Autodesk Inventor part; units mm, degrees
ref_plane "YZ Plane" through (0, 0, 0) normal (1, 0, 0) x (0, 1, 0)
ref_plane "XZ Plane" through (0, 0, 0) normal (0, 1, 0) x (-1, 0, 0)
ref_plane "XY Plane" through (0, 0, 0) normal (0, 0, 1) x (1, 0, 0)
sketch "Sketch1" plane through (0, 0, 0) normal (0, 0, 1) x (1, 0, 0)
  line L0 (-33.5517, 0) -> (33.5517, 0)
  line L1 (0, 0) -> (0, 2.95)
  line L2 (0, 2.95) -> (1, 2.95)
  line L3 (1, 2.95) -> (1, 2.5)
  line L4 (1, 2.5) -> (6.1, 2.5)
  arc A0 (8.6, 0) -> (6.1, 2.5) centre (6.1, 0) ccw
  line L5 (8.6, 0) -> (0, 0)
  dimension "d1" = 2.95
  dimension "d2" = 1
  dimension "d3" = 5
  dimension "d4" = 8.6
  dimension "d5" = 2.5
revolve "Revolution1" add sketch "Sketch1" angle 360 about axis through (-33.5517, 0, 0) along (1, 0, 0)
sketch "Sketch2" plane through (0, 0, 0) normal (-1, 0, 0) x (0, 0, 1)
  circle A0 centre (0, 0) radius 2.95
  line L0 (-0.25, 1.52) -> (0.25, 1.52)
  line L1 (0.25, 1.52) -> (0.25, 1.02)
  line L2 (0.25, 1.02) -> (-0.25, 1.02)
  line L3 (-0.25, 1.02) -> (-0.25, 1.52)
  line L4 (-0.25, -1.02) -> (0.25, -1.02)
  line L5 (0.25, -1.02) -> (0.25, -1.52)
  line L6 (0.25, -1.52) -> (-0.25, -1.52)
  line L7 (-0.25, -1.52) -> (-0.25, -1.02)
  line L8 (-0.25, 1.27) -> (0.25, 1.27) construction
  line L9 (-0.25, -1.27) -> (0.25, -1.27) construction
  point P0 (0, 1.52)
  point P1 (0, -1.02)
  dimension "d7" = 0.5
  dimension "d8" = 0.5
  dimension "d9" = 1.27
  dimension "d10" = 1.27
extrude "Extrusion1" add sketch "Sketch2" along normal blind 22.6 contours L0 L1 L2 L3 | L4 L5 L6 L7
sketch "Sketch4" plane through (0, 0, 0) normal (-1, 0, 0) x (0, 0, 1)
  line L0 (-0.25, 1.52) -> (0.25, 1.52)
  circle A0 centre (0, 0) radius 2.95
  circle A1 centre (0, 0) radius 2.5
  line L1 (-1.566, 2.5) -> (1.566, 2.5)
  point P0 (0, 2.5)
extrude "Extrusion2" cut sketch "Sketch4" against normal through all contours L1 A0 picked at (-0.846, 2.5951)
sketch "Sketch3" plane through (-22.6, 0, 0) normal (-1, 0, 0) x (0, 0, 1)
  line L0 (0.25, 1.52) -> (0.25, 1.02)
  line L1 (-0.25, 1.52) -> (0.25, 1.52)
  line L2 (-0.25, 1.02) -> (-0.25, 1.52)
  line L3 (0.25, 1.02) -> (-0.25, 1.02)
  line L4 (0.25, -1.02) -> (0.25, -1.52)
  line L5 (-0.25, -1.02) -> (0.25, -1.02)
  line L6 (-0.25, -1.52) -> (-0.25, -1.02)
  line L7 (0.25, -1.52) -> (-0.25, -1.52)
  point P0 (0, 0)
  point P1 (0, 1.27)
  point P2 (0, -1.27)
  point P3 (-0.25, 1.27)
  point P4 (-0.25, -1.27)
equation "\"d10\" = d9"
equation "\"Lead_solder\" = 1"
properties part number "LED 5mm Red height 1-20mm"
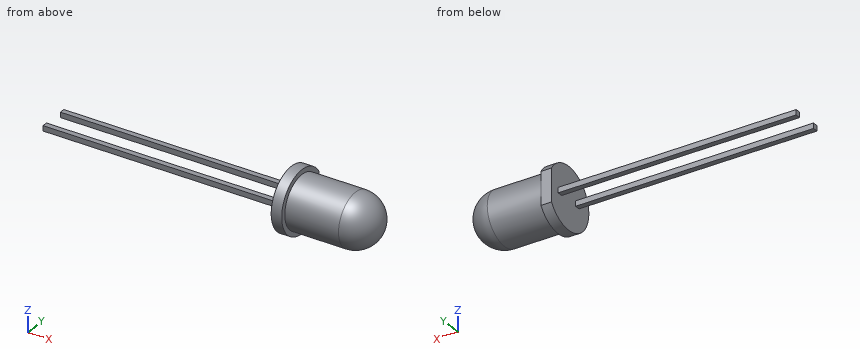
Source: CAD feature listing. Evaluate the final solid. Frame: model axes, mm. Round coordinates to 2 decimals unless told otherwise and drop trailing zeros. Order: outer loops, then holes, each group sorted by start corner. A loop starts at its lowest first (then second) coordinate and runs counter-clockwise, first axis right, second up. Notation, with made-up numbers: (-36.5, 42) -> (-15.5, 42) arc R9 ccw to (-15.5, 46) -> close; hole circle Ø5 at (40, 35.25). An arc over 180 degrees is marked (long way). Answer as CSV lines item,"result".
Item 1: Line query: L1, parallel to Z at x = -17, y = 1.35; L2, parallel to Y at x = 5, z = 0.95; L3, parallel to X at y = -1.6, z = -0.25. Output: solid intervals per line, ascending.
A:
L1,"-0.25 to 0.25"
L2,"-2.31 to 2.31"
L3,"0 to 8"
Item 2: Section A-A, the plane y = 0. Return loops of the section in (x, z).
A:
outline,"(0, -2.95) -> (1, -2.95) -> (1, -2.5) -> (6.1, -2.5) arc R2.5 ccw to (6.1, 2.5) -> (1, 2.5) -> (1, 2.95) -> (0, 2.95) -> close"
Item 3: Section D-D, the plane x = 3. Return loops of the section in (y, z), plus the area to 3 significant figures.
A:
outline,"circle Ø5 at (0, 0)"
area,"19.6 mm²"
Item 4: Section C-C, the plane z = -1.15. Return loops of the section in (x, y).
A:
outline,"(0, -2.72) -> (1, -2.72) -> (1, -2.22) -> (6.1, -2.22) arc R2.22 ccw to (6.1, 2.22) -> (1, 2.22) -> (1, 2.5) -> (0, 2.5) -> close"
Item 5: Pin query (flat end, axial travel): pin 1 Ø1 at (y, z) = (-1, -2) entering from +X; pin 2 Ø0.6 at (x, z) = (-14.5, 0) entering from -Y; pin 3 Ø0.6 at (x, y) = (-16.5, -1) entering from -Z. Return the tip coordinate at first contact, or that it passes through.
A:
pin 1,"x = 7.9"
pin 2,"y = -1.52"
pin 3,"z = -0.25"
Item 6: Section B-B, the plane x = -19.5. Return loops of the section in (y, z), plus the area to 3 significant figures.
A:
outline,"(-1.52, -0.25) -> (-1.02, -0.25) -> (-1.02, 0.25) -> (-1.52, 0.25) -> close; (1.02, -0.25) -> (1.52, -0.25) -> (1.52, 0.25) -> (1.02, 0.25) -> close"
area,"0.500 mm²"
